Geometry: see drawing. Coordinates: mm, zero at the bounding-box minimum. A direction names the side the tool comes from. Round coordinates to 2 decimals unless told otherwise and drop trailing zeros. Order: outer loops, then holes, each group sorted by start corner. A loop starts at its lowest first (then second) coordinate and runs counter-clockwise, first axis right, second up. Notation, with made-up numbers: M 37,-15.75 L 46,-15.75 A26 ccw 46,15.25 Z; hole C -32,-2.75 d5. An arc over 180 degrees is marked long. Answer in a Markdown table with one row per item. Add a question column.
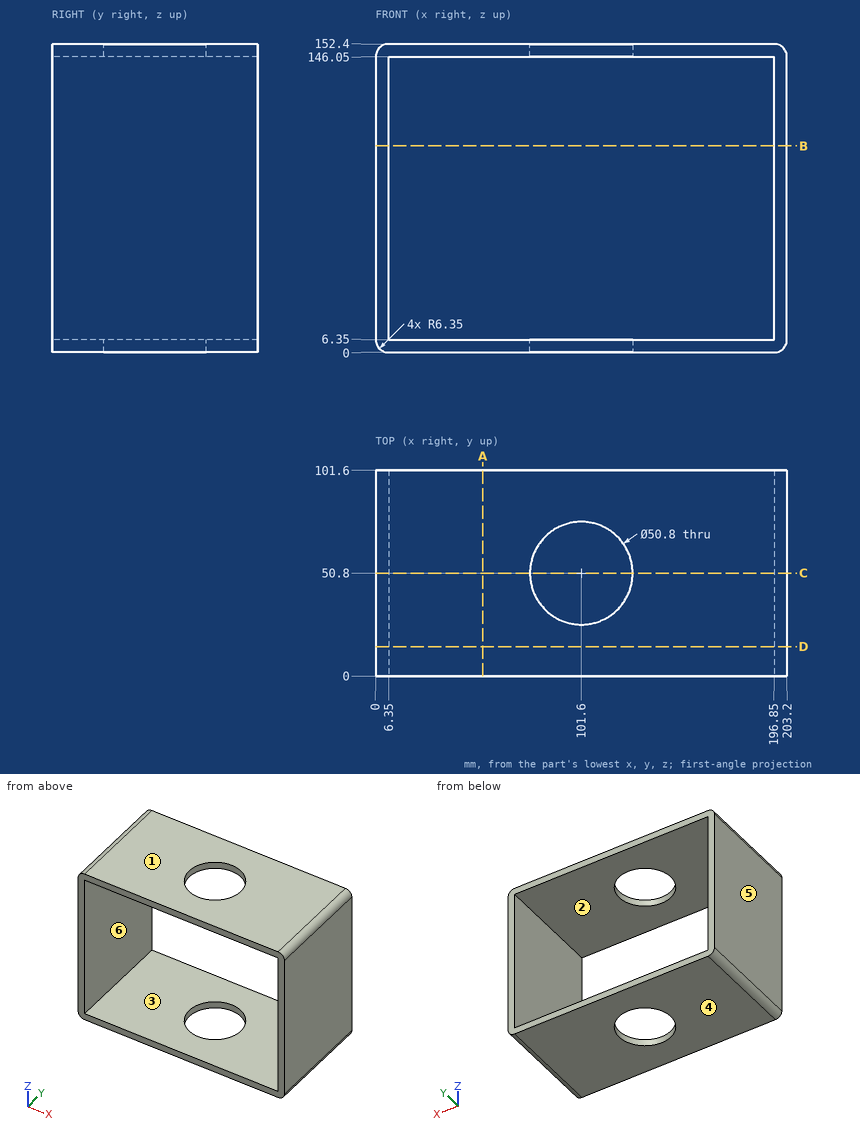
(1) Draft query along Z for the marked faces 1, 2, 3 and 4. Return one class per face: +Z half, -Z half, draft (parallel to the pull), parting line (faces both ways), or undercut.
(2) Line query: line 1 (X direction, y = 82.5, z = 67.5); line 2 (Z direction, x = 119.5, y = 13). Output: solid intervals per line, ascending. Write a range as from..to.
(3) Cut plane B-B (z = 102). Return loops of the section in (x, y).
(4) Access query for the marked faces 5 and 6. Directions: +Z, -Z, +X, -X, +Y, -Y. A direction counts if a zero-diameter tool reaches every point of the face in a straight line with its end or side. Return the directions, or none.
(5) Pin query (flat end, axial travel): pin 1 (6 mm diameter, centred on y = 83, z = 132.5, fed in from -X). Return the tip coordinate at first contact, or that it passes through.
(6) Cut plane A-A (x = 53). Return loops of the section in (y, z), and give its area (3 significant figures).
(7) Cut plane D-D (y = 14.5). Return loops of the section in (x, z), and give its area (3 significant figures).
(8) Cut plane C-C (y = 50.8). Return loops of the section in (x, z), and give its area (3 significant figures).
Answer list:
| question | item | result |
|---|---|---|
| 1 | face 1 | +Z half |
| 1 | face 2 | undercut |
| 1 | face 3 | undercut |
| 1 | face 4 | -Z half |
| 2 | line 1 | 0..6.35, 196.85..203.2 |
| 2 | line 2 | 0..6.35, 146.05..152.4 |
| 3 | outline | M 0,0 L 6.35,0 L 6.35,101.6 L 0,101.6 Z; M 196.85,0 L 203.2,0 L 203.2,101.6 L 196.85,101.6 Z |
| 4 | face 5 | +Z, -Z, -X, +Y, -Y |
| 4 | face 6 | +Y, -Y |
| 5 | pin 1 | x = 0 |
| 6 | outline | M 0,0 L 101.6,0 L 101.6,6.35 L 0,6.35 Z; M 0,146.05 L 101.6,146.05 L 101.6,152.4 L 0,152.4 Z |
| 6 | area | 1,290 mm² |
| 7 | outline | M 0,6.35 A6.35 ccw 6.35,0 L 196.85,0 A6.35 ccw 203.2,6.35 L 203.2,146.05 A6.35 ccw 196.85,152.4 L 6.35,152.4 A6.35 ccw 0,146.05 Z; hole M 6.35,6.35 L 196.85,6.35 L 196.85,146.05 L 6.35,146.05 Z |
| 7 | area | 4,320 mm² |
| 8 | outline | M 0,6.35 A6.35 ccw 6.35,0 L 76.2,0 L 76.2,6.35 L 6.35,6.35 L 6.35,146.05 L 76.2,146.05 L 76.2,152.4 L 6.35,152.4 A6.35 ccw 0,146.05 Z; M 127,0 L 196.85,0 A6.35 ccw 203.2,6.35 L 203.2,146.05 A6.35 ccw 196.85,152.4 L 127,152.4 L 127,146.05 L 196.85,146.05 L 196.85,6.35 L 127,6.35 Z |
| 8 | area | 3,680 mm² |
